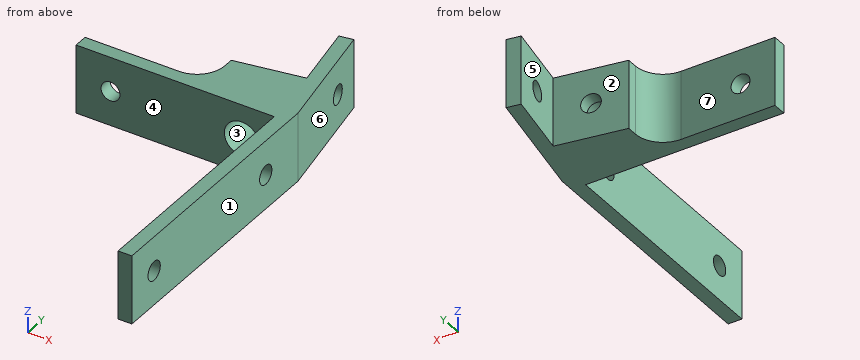
from build123d import *

# Parameters (mm, degrees)
BOSS_EXTRUDE1_DEPTH = 20
CUT_EXTRUDE5_REACH  = 126.766
SKETCH6_R           = 2.74999595
CUT_EXTRUDE10_REACH = 133.489
SKETCH11_R          = 2.75
CUT_EXTRUDE11_REACH = 100.344
SKETCH12_R          = 2.75
SKETCH13_R          = 2.75
CUT_EXTRUDE12_DEPTH = 4
CUT_EXTRUDE13_REACH = 99.421
SKETCH14_R          = 5


with BuildPart() as part:
    # Sketch1 → Boss-Extrude1 (new body)
    with BuildSketch(Plane.XY):
        with BuildLine():
            Line((0, 74.379660875), (-6.077686218, 108.84793223))
            Line((-6.077686218, 108.84793223), (-10.01691723, 108.153339519))
            Line((-10.01691723, 108.153339519), (-6.543953677, 88.457184459))
            Line((-6.543953677, 88.457184459), (-26.240108737, 84.984220906))
            Line((-26.240108737, 84.984220906), (-26.240108737, 81.999969263))
            ThreePointArc((-26.240108737, 81.999969263), (-28.583254488, 76.343115014), (-34.240108737, 73.999969263))
            Line((-34.240108737, 73.999969263), (-61.608001, 73.999969263))
            Line((-61.608001, 73.999969263), (-61.608001, 69.999969263))
            Line((-61.608001, 69.999969263), (-4, 69.999969263))
            Line((-4, 69.999969263), (-4, 0))
            Line((-4, 0), (0, 0))
            Line((0, 0), (0, 74.379660875))
        make_face()
    extrude(amount=BOSS_EXTRUDE1_DEPTH)

    # Sketch6 → Cut-Extrude5 (cut, up to next)
    with BuildSketch(Plane.ZY.offset(4), mode=Mode.PRIVATE) as cut_extrude5_sk1:
        with Locations((9.9999995, 59.999977673)):
            Circle(SKETCH6_R)
    cut_extrude5_tool1 = extrude(cut_extrude5_sk1.sketch, amount=-CUT_EXTRUDE5_REACH, mode=Mode.PRIVATE) & part.part
    # Sketch6 → Cut-Extrude5 (cut, up to next)
    with BuildSketch(Plane.ZY.offset(4), mode=Mode.PRIVATE) as cut_extrude5_sk2:
        with Locations((9.9999995, 9.999962864)):
            Circle(SKETCH6_R)
    cut_extrude5_tool2 = extrude(cut_extrude5_sk2.sketch, amount=-CUT_EXTRUDE5_REACH, mode=Mode.PRIVATE) & part.part
    add(cut_extrude5_tool1.solids().sort_by_distance((-4, 59.999978, 9.999999))[0], mode=Mode.SUBTRACT)
    add(cut_extrude5_tool2.solids().sort_by_distance((-4, 9.999963, 9.999999))[0], mode=Mode.SUBTRACT)

    # Sketch11 → Cut-Extrude10 (cut, up to next)
    with BuildSketch(Plane(origin=(12.719671136, 2.242821207, 0), x_dir=(0, 0, -1), z_dir=(0.9848077530122074, 0.1736481776669349, 0)), mode=Mode.PRIVATE) as cut_extrude10_sk1:
        with Locations(Location((-10, 98.249666696, 0), (0, 0, 90))):
            Circle(SKETCH11_R)
    cut_extrude10_tool1 = extrude(cut_extrude10_sk1.sketch, amount=-CUT_EXTRUDE10_REACH, mode=Mode.PRIVATE) & part.part
    add(cut_extrude10_tool1.solids().sort_by_distance((-4.341204, 98.999855, 10))[0], mode=Mode.SUBTRACT)

    # Sketch12 → Cut-Extrude11 (cut, up to next)
    with BuildSketch(Plane(origin=(0, 73.999969263, 0), x_dir=(1, 0, 0), z_dir=(0, 1, 0)), mode=Mode.PRIVATE) as cut_extrude11_sk1:
        with Locations(Location((-51.608001, -10, 0), (0, 0, 270))):
            Circle(SKETCH12_R)
    cut_extrude11_tool1 = extrude(cut_extrude11_sk1.sketch, amount=-CUT_EXTRUDE11_REACH, mode=Mode.PRIVATE) & part.part
    add(cut_extrude11_tool1.solids().sort_by_distance((-51.608001, 73.999969, 10))[0], mode=Mode.SUBTRACT)

    # Sketch13 → Cut-Extrude12 (cut)
    with BuildSketch(Plane(origin=(-15.324393801, 86.908955963, 0), x_dir=(0.9848077530122072, 0.17364817766693516, 0), z_dir=(-0.1736481776669352, 0.9848077530122074, 0))):
        with Locations(Location((-1.084107434, -10, 0), (0, 0, 180))):
            Circle(SKETCH13_R)
    extrude(amount=-CUT_EXTRUDE12_DEPTH, mode=Mode.SUBTRACT)

    # Cut-Extrude13: up to this plane
    cut_extrude13_end = Plane(origin=(-4, 69.999969263, 20), z_dir=(0, -1, 0))
    # Sketch14 → Cut-Extrude13 (cut, up to the surface)
    with BuildSketch(Plane(origin=(-14.629801091, 82.969724951, 0), x_dir=(0.9848077530122072, 0.17364817766693522, 0), z_dir=(-0.17364817766693524, 0.9848077530122074, 0)), mode=Mode.PRIVATE) as cut_extrude13_sk1:
        with Locations(Location((-1.084107434, -10, 0), (0, 0, 180))):
            Circle(SKETCH14_R)
    cut_extrude13_tool1 = split(extrude(cut_extrude13_sk1.sketch, amount=-CUT_EXTRUDE13_REACH, mode=Mode.PRIVATE), bisect_by=cut_extrude13_end, keep=Keep.BOTH, mode=Mode.PRIVATE)
    add(cut_extrude13_tool1.solids().sort_by_distance((-15.697438, 82.781472, 10))[0], mode=Mode.SUBTRACT)


solid = part.part
For this review, take the finished solid that the model builds, in its own axes (mm). Face numbers are marked on the shaded views. A direction names the side the tool comes from. Give positions to 0.01 mm unless a question says otherwise; leave off trailing zeros. Order: outer loops, then holes, each group sorted by start corner. A loop starts at its lowest first (then second) coordinate and runs counter-clockwise, first axis right, second up. Notation, with made-up numbers: (-36, 87.25) - (-18, 87.25) arc R34 ccw to (-18, 122.25) - close; hole circle Ø1 at (-4, 24). An arc over 180 degrees is marked (long way). Answer as a JSON object with one key per item and string values. Group by question number.
Item 1: Take a section at D-D on y = 50. Give the boundary of the cut face in (x, z).
Item 2: Take a section at B-B on x = -56. Give the boundary of the cut face in (y, z), and give its area (3 significant figures).
Item 3: Machinability: for the marked faces 4, 5, 6 and 7, which of the approach directions +Z, -Z, +X, -X, +Y, -Y give a long, thin tool a straight path to every point of the face, cutting with its end or side? Answer none if there is none.
Item 4: Take a section at C-C on z = 10. Give the number of separate pieces and of enclosed holes in the cut face, and give its area (3 significant figures).
Item 5: Clearance check with flat-ended pins moving along their axes: pin 1 Ø5 at (x, z) = (-51.61, 10) entering from +Y; pin 2 Ø1.5 at (y, z) = (84, 11.5) entering from -X; pin 3 Ø10 at (x, z) = (-25.5, 5) entering from -Y; pin 4 Ø10 at (y, z) = (86.5, 8) entering from +X. State where each tip first meets the part, or that it passes through.
Item 6: Take a section at A-A on z = 1.5. Give the boundary of the cut face in (x, y).
Item 7: Draft analysis for pull direction X (two halves, no side actions). For the marked faces 1, 2 and 3, state which applies: pulls with the +X half, pulls with the -X half, needs draft (parallel to the pull), parting line crosses it, or undercut.
Item 8: Wall thickness on line 1 along X through (y, z) = (71.9, 10); line 2 along Y through (x, z) = (-36, 18); line 3 along X through (y, z) = (6, 9.75): over which ranges is each line inside the solid? List them lowest first.
Reported:
{
 "1": {"outline": "(-4, 0) - (0, 0) - (0, 20) - (-4, 20) - close"},
 "2": {"outline": "(70, 0) - (74, 0) - (74, 20) - (70, 20) - close", "area": "80.0 mm^2"},
 "3": {"face 4": "+Z, -Z, -X, -Y", "face 5": "+Z, -Z, -X", "face 6": "+Z, -Z, +X, +Y", "face 7": "+Z, -Z, -X, +Y"},
 "4": {"separate pieces": "6", "enclosed holes": "0", "area": "709 mm^2"},
 "5": {"pin 1": "through", "pin 2": "x = -26.24", "pin 3": "y = 70", "pin 4": "x = -1.26"},
 "6": {"outline": "(-61.61, 70) - (-4, 70) - (-4, 0) - (0, 0) - (0, 74.38) - (-6.08, 108.85) - (-10.02, 108.15) - (-6.54, 88.46) - (-26.24, 84.98) - (-26.24, 82) arc R8 cw to (-34.24, 74) - (-61.61, 74) - close"},
 "7": {"face 1": "pulls with the +X half", "face 2": "pulls with the -X half", "face 3": "undercut"},
 "8": {"line 1": "-61.61 to -54.36, -48.86 to -18.86, -8.7 to 0", "line 2": "70 to 74", "line 3": "-4 to 0"}
}
